Autodesk Inventor part; units mm, degrees
ref_plane "工作平面1" through (10, 22, 0) normal (-0.3926, -0.6503, -0.6503) x (0.8561, 0, -0.5169)
ref_plane "YZ Plane" through (0, 0, 0) normal (1, 0, 0) x (0, 1, 0)
ref_plane "XZ Plane" through (0, 0, 0) normal (0, 1, 0) x (-1, 0, 0)
sketch "草圖1" plane through (0, 0, 0) normal (0, 1, 0) x (-1, 0, 0)
  line L0 (0, 0) -> (-63, 0)
  line L1 (-63, 0) -> (-63, -42)
  line L2 (-63, -42) -> (0, -42)
  line L3 (0, -42) -> (0, 0)
  dimension "d0" = 63
  dimension "d1" = 42
extrude "擠出1" add sketch "草圖1" along normal mid plane 44
sketch "草圖2" plane through (0, 22, 0) normal (0, 1, 0) x (1, 0, 0)
  line L0 (0, 0) -> (63, 0)
  line L1 (10, 0) -> (63, 12)
  line L2 (63, 0) -> (63, 42)
  dimension "d4" = 10
  dimension "d5" = 30
extrude "擠出2" cut sketch "草圖2" against normal blind 60
sketch "草圖3" plane through (63, -22, -42) normal (1, 0, 0) x (0, 0, -1)
  line L0 (-30, 24) -> (-10, 44)
  line L1 (0, 44) -> (-42, 44)
  line L2 (-30, 44) -> (-30, 0)
  point P0 (-42, 22)
  point P1 (-30, 2)
  dimension "d8" = 20
  dimension "d9" = 20
ref_plane "工作平面1" through (10, 22, 0) normal (-0.3926, -0.6503, -0.6503) x (0.8561, 0, -0.5169)
sketch "草圖4" plane through (10, 22, 0) normal (-0.3926, -0.6503, -0.6503) x (0.8561, 0, -0.5169)
  line L0 (-15.1543, -12.3218) -> (93.717, -12.3218)
  line L1 (93.717, -12.3218) -> (93.717, 28.8166)
  line L2 (93.717, 28.8166) -> (-15.1543, 28.8166)
  line L3 (-15.1543, 28.8166) -> (-15.1543, -12.3218)
  point P0 (-8.5606, 13.3512)
extrude "擠出3" cut sketch "草圖4" against normal blind 40
mirror "鏡射1" about plane through (0, 0, 0) normal (0, 1, 0) of "擠出3"
properties part number "59"
Input: part model. Units: mm. Frame: model coordinates. Give positions to 0.01 mm unless a question says otherwise; leave off trailing zeros. Write each loop counter-clockwise with the first axis right and the second up, starting at its lowest first coordinate (ties: lowest second). Pieces come first, ordered by that corner, then holes. Notation, with made-up numbers: (-21.5, 36) - (28.5, 36) arc R20 ccw to (28.5, 47) - close; hole circle Ø7 at (-2.75, 83). An arc over 180 degrees is marked (long way). Write item = value, one per line. Start each with the question number.
1. Section query A-A, the plane y = 1. Output: boundary loops of the cut face in (x, z), then the cut area to 3 significant figures.
2. First-contact query: pin 1 Ø10 at (y, z) = (4, -29) entering from -X; pin 2 Ø5 at (x, z) = (44.5, -16) entering from -Y; pin 3 Ø1 at (x, y) = (18.5, 6.5) entering from +Z; pin 4 Ø2 at (x, y) = (33.5, 14.5) entering from +Z. Flat tips, straight axial feed; report the tip coordinate or a pass-through.
3. Ray query, L1, parallel to Y at x = 31.5, z = -5; L2, parallel to Z at x = 46, y = 18; L3, parallel to Z at x = 53.5, y = -18.5. Return the intervals inside material, ascending.
4. Section query B-B, the plane z = -20.5. Output: boundary loops of the cut face in (x, y).
5. Section query C-C, the plane x = 44. Output: boundary loops of the cut face in (y, z).
Check sheet entries:
q1.outline = (0, -42) - (63, -42) - (63, -12) - (10, 0) - (0, 0) - close
q1.area = 2,330 mm2
q2.pin_1 = 0
q2.pin_2 = -20.09
q2.pin_3 = -1.81
q2.pin_4 = -5.52
q3.L1 = -14.02 to 14.02
q3.L2 = -42 to -17.74
q3.L3 = -42 to -22.76
q4.outline = (0, -22) - (43.95, -22) - (63, -10.5) - (63, 10.5) - (43.95, 22) - (0, 22) - close
q5.outline = (-22, -42) - (22, -42) - (22, -20.53) - (9.17, -7.7) - (-9.17, -7.7) - (-22, -20.53) - close
